Could you check a few things on this model? Use its own coordinates, in mm. Face numbers are marked on the shaded views. A direction names the side the tool comes from. Coordinates: 2 decimals unless noted, no trailing zeros. Order: outer loops, then holes, each group sorted by start corner. A loop starts at its lowest first (then second) coordinate and runs counter-clockwise, first axis right, second up. Notation, with made-up numbers: (4.25, 24.25) -> (44.25, 24.25) arc R26 ccw to (44.25, 63.25) -> close; hole circle Ø1 at (15.5, 23.25). An arc over 180 degrees is marked (long way). Put each result on its own line as item: value. Start each with the question number.
Q1. If we section it at C-C (x = 43.5): Please give me the cut outline in (y, z), and give its area (3 significant figures).
Q2. If we section it at D-D (z = 35): Please give me the cut outline in (x, y), and give its area (3 significant figures).
Q3. Please list where these lines run through material, in increasing order: line 1 along X through (y, z) = (-366, 16); line 2 along X through (y, z) = (-130, 41.5); line 3 along Y through (x, z) = (85, -7.5).
Q4. Will these pins go through, and if not, where does the flat tip stop? pin 1 (10 mm diameter, centred on x = 208.5, z = 5.5, fed in from -Y); pin 2 (15 mm diameter, centred on y = -326.5, z = 7.5, fed in from +X); pin 3 (3 mm diameter, centred on x = 177.5, z = -3, fed in from -Y); pin 4 (6 mm diameter, centred on y = 29.5, z = 9, fed in from +X).
Q5. If we section it at A-A (y = -370): Please give me the cut outline in (x, z).
Q6. If we section it at B-B (z = -14): Please give me the cut outline in (x, y), and give its area (3 significant figures).
Q7. For the marked faces 1, 2, 3, 4 and 5, which set-ups out of +Z, -Z, +X, -X, +Y, -Y let a thin tool reach every point of the face, with its end or its side?
from build123d import *

# Parameters (mm, degrees)
F1_DEPTH = 20
F2_W     = 20
F2_H     = 495
F3_DEPTH = 60
F4_DEPTH = 30
F5_DEPTH = 20


with BuildPart() as f1:
    # F0 (on Top) → F1 (new body)
    with BuildSketch(Plane.XY):
        Polygon((120, 40), (20, 40), (0, 20), (0, 0), (120, 0), align=None)
        Polygon((220, 40), (120, 40), (120, 0), (240, 0), (240, 20), align=None)
    extrude(amount=-F1_DEPTH)

    # F2 (on Top) → F3 (join)
    with BuildSketch(Plane.XY):
        with Locations((110, -207.5)):
            Rectangle(F2_W, F2_H)
    extrude(amount=F3_DEPTH)

    # F2 (on Top) → F4 (join)
    with BuildSketch(Plane.XY):
        Polygon((140, 40), (120, 40), (120, -455), (140, -455), (140, -110), align=None)
    extrude(amount=F4_DEPTH)

    # F2 (on Top) → F5 (join)
    with BuildSketch(Plane.XY):
        Polygon((200, 40), (140, 40), (140, -110), (200, 0), align=None)
    extrude(amount=F5_DEPTH)


solid = f1.part
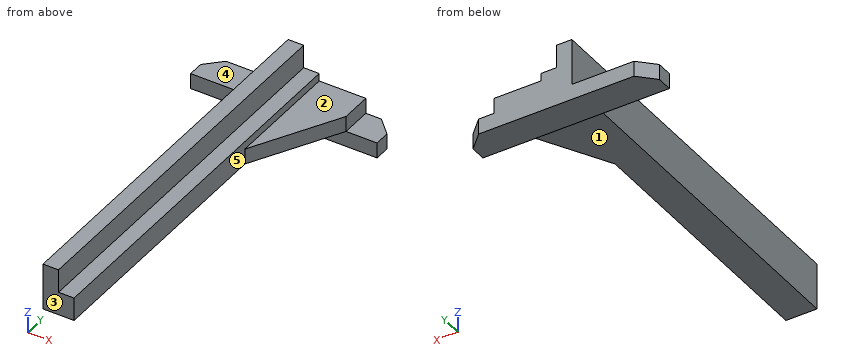
The answers:
1. outline: (0, -20) -> (40, -20) -> (40, 0) -> (0, 0) -> close
1. area: 800 mm^2
2. outline: (100, -455) -> (120, -455) -> (120, 40) -> (100, 40) -> close
2. area: 9,900 mm^2
3. line 1: 100 to 140
3. line 2: 100 to 120
3. line 3: 0 to 40
4. pin 1: through
4. pin 2: x = 140
4. pin 3: y = 0
4. pin 4: x = 200
5. outline: (100, 0) -> (140, 0) -> (140, 30) -> (120, 30) -> (120, 60) -> (100, 60) -> close
6. outline: (0, 0) -> (240, 0) -> (240, 20) -> (220, 40) -> (20, 40) -> (0, 20) -> close
6. area: 9,200 mm^2
7. face 1: -Z, +X, -X, -Y
7. face 2: +Z, +X, +Y, -Y
7. face 3: +Z, -Z, +X, -X, -Y
7. face 4: +Z, -X, +Y, -Y
7. face 5: +Z, +X, -Y
